from build123d import *

# Parameters (mm, degrees)
BOSS_EXTRUDE1_DEPTH = 5
SKETCH2_W           = 7.5
SKETCH2_H           = 50
BOSS_EXTRUDE2_DEPTH = 55
FILLET1_R           = 3
FILLET2_R           = 3
SKETCH3_R           = 1.5
SKETCH3_R_2         = 3.5
CUT_EXTRUDE1_DEPTH  = 83.006097334
SKETCH4_R           = 11.5
CUT_EXTRUDE2_DEPTH  = 3
SKETCH6_R           = 2
CUT_EXTRUDE3_DEPTH  = 66.383484153


with BuildPart() as part:
    # Sketch1 → Boss-Extrude1 (new body)
    with BuildSketch(Plane(origin=(0, 0, 0), x_dir=(1, 0, 0), z_dir=(0, 1, 0))):
        with BuildLine():
            Line((-25, 25), (20, 25))
            ThreePointArc((20, 25), (23.535533906, 23.535533906), (25, 20))
            Line((25, 20), (25, -20))
            ThreePointArc((25, -20), (23.535533906, -23.535533906), (20, -25))
            Line((20, -25), (-25, -25))
            Line((-25, -25), (-25, 25))
        make_face()
    extrude(amount=BOSS_EXTRUDE1_DEPTH)

    # Sketch2 → Boss-Extrude2 (add)
    with BuildSketch(Plane(origin=(0, 5, 0), x_dir=(1, 0, 0), z_dir=(0, 1, 0))):
        with Locations((-21.25, 0)):
            Rectangle(SKETCH2_W, SKETCH2_H)
    extrude(amount=BOSS_EXTRUDE2_DEPTH)

    # Fillet1
    fillet1_edges = [part.edges().sort_by_distance(p)[0] for p in [
        (-17.5, 5, 0),
    ]]
    fillet(fillet1_edges, radius=FILLET1_R)

    # Fillet2
    fillet2_edges = [part.edges().sort_by_distance(p)[0] for p in [
        (-25, 0, 0),
    ]]
    fillet(fillet2_edges, radius=FILLET2_R)

    # Sketch3 → Cut-Extrude1 (cut, through all)
    with BuildSketch(Plane.ZY.offset(25)):
        with Locations((15.5, 53)):
            Circle(SKETCH3_R)
        with Locations(Location((-15.5, 53, 0), (0, 0, 180))):
            Circle(SKETCH3_R)
        with Locations((0, 37.5)):
            Circle(SKETCH3_R_2)
        with Locations(Location((15.5, 22, 0), (0, 0, 180))):
            Circle(SKETCH3_R)
        with Locations((-15.5, 22)):
            Circle(SKETCH3_R)
    extrude(amount=-CUT_EXTRUDE1_DEPTH, mode=Mode.SUBTRACT)

    # Sketch4 → Cut-Extrude2 (cut)
    with BuildSketch(Plane(origin=(-17.5, 0, 0), x_dir=(0, 0, -1), z_dir=(1, 0, 0))):
        with Locations((0, 37.5)):
            Circle(SKETCH4_R)
    extrude(amount=-CUT_EXTRUDE2_DEPTH, mode=Mode.SUBTRACT)

    # Sketch6 → Cut-Extrude3 (cut, through all)
    with BuildSketch(Plane(origin=(0, 5, 0), x_dir=(1, 0, 0), z_dir=(0, 1, 0))):
        with Locations(Location((12, -10, 0), (0, 0, 270))):
            Circle(SKETCH6_R)
        with Locations(Location((-4, -10, 0), (0, 0, 270))):
            Circle(SKETCH6_R)
        with Locations(Location((12, 10, 0), (0, 0, 90))):
            Circle(SKETCH6_R)
        with Locations(Location((-4, 10, 0), (0, 0, 90))):
            Circle(SKETCH6_R)
    extrude(amount=-CUT_EXTRUDE3_DEPTH, mode=Mode.SUBTRACT)


solid = part.part
The listing builds one solid part. Answer for the finished solid, in the listing's coordinates (mm). A direction names the side the tool comes from. Coordinates: 2 decimals unless noted, no trailing zeros. Order: outer loops, then holes, each group sorted by start corner. A loop starts at its lowest first (then second) coordinate and runs counter-clockwise, first axis right, second up. Notation, with made-up numbers: M 52.25,-17.75 L 107.25,-17.75 A22 cw 107.25,16.25 Z; hole C 59,47.25 d7. An arc over 180 degrees is marked long. Use CSV: the item, a comma, the result in double quotes.
Q1. Straight lines are drawn through the part: L1, parallel to Y at x = -21.75, z = 15.5; L2, parallel to X at y = 2.65, z = 10; L3, parallel to X at y = 39, z = 3.5. For each, find the intervals that lie inside material, in ascending order.
Here are the results:
L1,"0 to 20.5, 23.5 to 51.5, 54.5 to 60"
L2,"-24.98 to -6, -2 to 10, 14 to 25"
L3,"-25 to -20.5"
Q2. Section A-A (z = 0) is taken. Determine the outline of the cut face in (x, y), then the cut area to 3 significant figures.
Here are the results:
outline,"M -25,3 A3 ccw -22,0 L 25,0 L 25,5 L -14.5,5 A3 cw -17.5,8 L -17.5,26 L -20.5,26 L -20.5,34 L -25,34 Z; M -25,41 L -20.5,41 L -20.5,49 L -17.5,49 L -17.5,60 L -25,60 Z"
area,"562 mm2"
Q3. A tool of negligible diameter and unlimited length cuts with its end or side. For faces 4 (the cylindrical face through (-23, 41, 0)), 5 (the flat face through (-20.5, 35, 3)), 6 (the flat face through (-17.5, 33.6, 11.5)), from which of +Z, -Z, +X, -X, +Y, -Y can it reach the whole face along a straight path? Write none if from no direction.
Here are the results:
face 4,"+X, -X"
face 5,"+X"
face 6,"+Z, -Z, +X, +Y"
Q4. Section C-C (z = -15.5) is taken. Determine the outline of the cut face in (x, y).
Here are the results:
outline,"M -25,3 A3 ccw -22,0 L 25,0 L 25,5 L -14.5,5 A3 cw -17.5,8 L -17.5,20.5 L -25,20.5 Z; M -25,23.5 L -17.5,23.5 L -17.5,51.5 L -25,51.5 Z; M -25,54.5 L -17.5,54.5 L -17.5,60 L -25,60 Z"
Q5. Section D-D (y = 53) is taken. Determine the outline of the cut face in (x, z).
Here are the results:
outline,"M -25,-25 L -17.5,-25 L -17.5,-17 L -25,-17 Z; M -25,-14 L -17.5,-14 L -17.5,14 L -25,14 Z; M -25,17 L -17.5,17 L -17.5,25 L -25,25 Z"
Q6. Determine the mould class of faces 1 (the cylindrical face through (24, 2, 23)), 2 (the cylindrical face through (10, 3, -10)), 3 (the flat face through (-18, 23, -25)) for opening direction Z: pulls with the +Z half, pulls with the -Z half, needs draft (parallel to the pull), parting line crosses it, or undercut.
Here are the results:
face 1,"pulls with the +Z half"
face 2,"undercut"
face 3,"pulls with the -Z half"
Q7. Given pin 1 Ø3.5 at (y, z) = (53, 15.5) entering from +X; pin 2 Ø2.5 at (y, z) = (22, 15.5) entering from -X; pin 3 Ø18.5 at (y, z) = (37.5, 0) entering from +X; pin 4 Ø4.5 at (x, z) = (-4, 10) entering from +Y, each flat-ended and moving along its own axis, determine where each tip first touches the part or whether it passes through.
Here are the results:
pin 1,"x = -17.5"
pin 2,"through"
pin 3,"x = -20.5"
pin 4,"y = 5"
Q8. Section B-B (x = -4) is taken. Determine the outline of the cut face in (y, z).
Here are the results:
outline,"M 0,-25 L 5,-25 L 5,-12 L 0,-12 Z; M 0,-8 L 5,-8 L 5,8 L 0,8 Z; M 0,12 L 5,12 L 5,25 L 0,25 Z"
